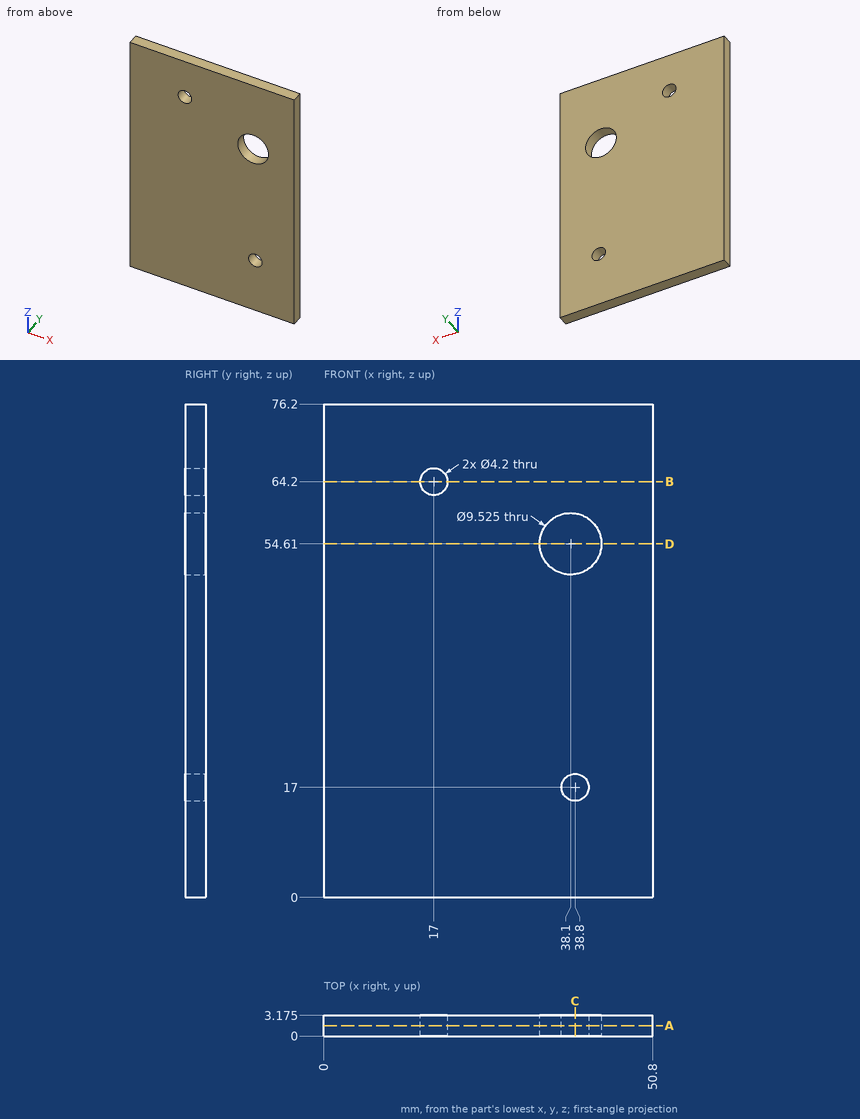
Part print with two shaded views. Sizes in mm from the minimum x, y, z corner. Coordinates: 2 decimals unless noted, no trailing zeros. Order: outer loops, then holes, each group sorted by start corner. A loop starts at its lowest first (then second) coordinate and runs counter-clockwise, first axis right, second up.
(1) Saw through at C-C, the plane x = 38.8. Write the cut outline in (y, z) (3 decimals).
Solution:
outline: (0, 0) - (3.175, 0) - (3.175, 14.9) - (0, 14.9) - close; (0, 19.1) - (3.175, 19.1) - (3.175, 49.899) - (0, 49.899) - close; (0, 59.321) - (3.175, 59.321) - (3.175, 76.2) - (0, 76.2) - close
(2) Saw through at A-A, the plane y = 1.6. Write the cut outline in (x, z) (1 decimal), and give its area (3 significant figures).
Solution:
outline: (0, 0) - (50.8, 0) - (50.8, 76.2) - (0, 76.2) - close; hole circle Ø4.2 at (17, 64.2); hole circle Ø9.5 at (38.1, 54.6); hole circle Ø4.2 at (38.8, 17)
area: 3,770 mm2
(3) Saw through at D-D, the plane z = 54.61. Write the cut outline in (x, y) (1 decimal).
Solution:
outline: (0, 0) - (33.3, 0) - (33.3, 3.2) - (0, 3.2) - close; (42.9, 0) - (50.8, 0) - (50.8, 3.2) - (42.9, 3.2) - close
(4) Saw through at B-B, the plane z = 64.2. Write the cut outline in (x, y) (3 decimals), and give its area (3 significant figures).
Solution:
outline: (0, 0) - (14.9, 0) - (14.9, 3.175) - (0, 3.175) - close; (19.1, 0) - (50.8, 0) - (50.8, 3.175) - (19.1, 3.175) - close
area: 148 mm2
(5) Pin check, flat tip, straight feed: pin 1 Ø4 at (x, z) = (38.8, 17) entering from -Y (3 decimals). Stop position of the tip, or through.
Solution:
pin 1: passes through
(6) Drill centre lines: L1, parallel to X at y = 2.1, z = 54.61; L2, parallel to Z at x = 38.8, y = 1.75; L3, parallel to Z at x = 17, y = 0.95. Where is each one in solid material? Low to high.
Solution:
L1: x = 0 to 33.34, 42.86 to 50.8
L2: z = 0 to 14.9, 19.1 to 49.9, 59.32 to 76.2
L3: z = 0 to 62.1, 66.3 to 76.2
